For this review, take the finished solid that the model builds, in its own axes (mm). Give positions to 0.01 mm unless a question says otherwise; leave off trailing zeros. Write each loop counter-clockwise with the first axis right and the second up, starting at its lowest first coordinate (ties: lowest second). Pieces come first, ordered by that corner, then holes.
1) For P1, Ø3, axis at x = 0, z = 142.5, coming from the +Y side; P2, Ø2.5, axis at x = 0, z = 142.5, coming from the -Y side, all flat-tipped, find the tip position at first contact; note any pin that passes through.
2) We need section A-A on z = 57. Give the boundary of the cut face in (x, y), and give its area (3 significant figures).
3) Wall thickness on line 1 along X through (y, z) = (1.2, 67.5); line 2 along X through (y, z) = (-0.75, 127.5); line 3 along Y through (x, z) = (3.25, 81): over which ranges is each line inside the solid? List them lowest first.
from build123d import *

# Parameters (mm, degrees)
EXTRUDE1_DEPTH             = 150
SKETCH2_R                  = 1.2
EXTRUDE2_DEPTH             = 4.8
SKETCH_R                   = 2.1
SKETCH_R_2                 = 1.2
EXTRUDE4_DEPTH             = 2.3
CHAMFER1_SIZE              = 0.2
LPATTERN1_COUNT            = 10
LPATTERN1_PITCH            = 15
CHAMFER1_OF_LPATTERN1_SIZE = 0.2


with BuildPart() as part:
    # Sketch1 → Extrude1 (new body)
    with BuildSketch(Plane.XY):
        with BuildLine():
            Line((-3.3, -2.4), (3.3, -2.4))
            Line((3.3, -2.4), (3.5, -2.2))
            Line((3.5, -2.2), (3.5, 0.106274607))
            ThreePointArc((3.5, 0.106274607), (3.091294745, 0.282570681), (2.840065792, 0.65))
            Line((2.840065792, 0.65), (2.340065792, 0.65))
            Line((2.340065792, 0.65), (2.340065792, 1.15))
            Line((2.340065792, 1.15), (2.840065792, 1.15))
            ThreePointArc((2.840065792, 1.15), (3.091294745, 1.517429319), (3.5, 1.693725393))
            Line((3.5, 1.693725393), (3.5, 2.2))
            Line((3.5, 2.2), (3.3, 2.4))
            Line((3.3, 2.4), (-3.3, 2.4))
            Line((-3.3, 2.4), (-3.5, 2.2))
            Line((-3.5, 2.2), (-3.5, 1.693725393))
            ThreePointArc((-3.5, 1.693725393), (-3.091294745, 1.517429319), (-2.840065792, 1.15))
            Line((-2.840065792, 1.15), (-2.340065792, 1.15))
            Line((-2.340065792, 1.15), (-2.340065792, 0.65))
            Line((-2.340065792, 0.65), (-2.840065792, 0.65))
            ThreePointArc((-2.840065792, 0.65), (-3.091294745, 0.282570681), (-3.5, 0.106274607))
            Line((-3.5, 0.106274607), (-3.5, -2.2))
            Line((-3.5, -2.2), (-3.3, -2.4))
        make_face()
    extrude(amount=EXTRUDE1_DEPTH)

    # Sketch2 → Extrude2 (cut)
    with BuildSketch(Plane(origin=(0, 2.4, 0), x_dir=(1, 0, 0), z_dir=(0, 1, 0))):
        with Locations((0, -7.5)):
            Circle(SKETCH2_R)
    extrude2 = extrude(amount=-EXTRUDE2_DEPTH, mode=Mode.SUBTRACT)

    # Sketch → Extrude4 (cut)
    with BuildSketch(Plane(origin=(0, 2.4, 0), x_dir=(1, 0, 0), z_dir=(0, 1, 0))):
        with Locations((0, -7.5)):
            Circle(SKETCH_R)
        with Locations((0, -7.5)):
            Circle(SKETCH_R_2, mode=Mode.SUBTRACT)
    extrude4 = extrude(amount=-EXTRUDE4_DEPTH, mode=Mode.SUBTRACT)

    # Chamfer1
    chamfer1_edges = [part.edges().sort_by_distance(p)[0] for p in [
        (-1.2, -2.4, 7.5),
        (-2.1, 2.4, 7.5),
    ]]
    chamfer(chamfer1_edges, length=CHAMFER1_SIZE)

    # LPattern1: Extrude2, Extrude4 ×10
    with Locations(*[(0, 0, i * LPATTERN1_PITCH) for i in range(1, LPATTERN1_COUNT)]):
        add(extrude2, mode=Mode.SUBTRACT)
        add(extrude4, mode=Mode.SUBTRACT)

    # Chamfer1 of LPattern1
    chamfer1_of_lpattern1_edges = [part.edges().sort_by_distance(p)[0] for p in [
        (-1.2, -2.4, 22.5),
        (-2.1, 2.4, 22.5),
        (-1.2, -2.4, 37.5),
        (-2.1, 2.4, 37.5),
        (-1.2, -2.4, 52.5),
        (-2.1, 2.4, 52.5),
        (-1.2, -2.4, 67.5),
        (-2.1, 2.4, 67.5),
        (-1.2, -2.4, 82.5),
        (-2.1, 2.4, 82.5),
        (-1.2, -2.4, 97.5),
        (-2.1, 2.4, 97.5),
        (-1.2, -2.4, 112.5),
        (-2.1, 2.4, 112.5),
        (-1.2, -2.4, 127.5),
        (-2.1, 2.4, 127.5),
        (-1.2, -2.4, 142.5),
        (-2.1, 2.4, 142.5),
    ]]
    chamfer(chamfer1_of_lpattern1_edges, length=CHAMFER1_OF_LPATTERN1_SIZE)


solid = part.part
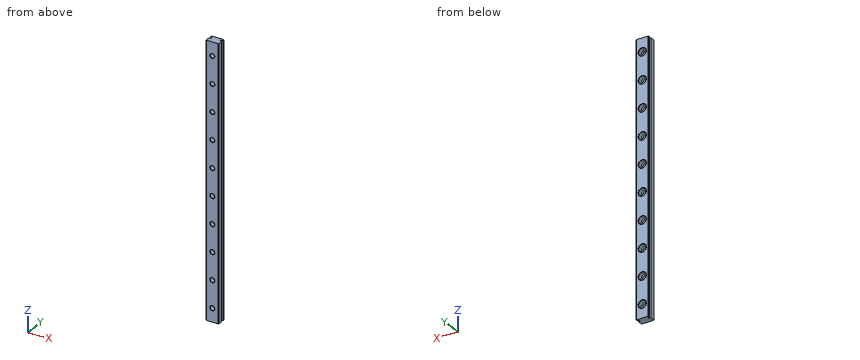
Results list:
1. P1: stops at y = 0.1
1. P2: stops at y = -2.25
2. outline: (-3.5, -2.2) - (-3.3, -2.4) - (3.3, -2.4) - (3.5, -2.2) - (3.5, 0.11) arc R0.8 cw to (2.84, 0.65) - (2.34, 0.65) - (2.34, 1.15) - (2.84, 1.15) arc R0.8 cw to (3.5, 1.69) - (3.5, 2.2) - (3.3, 2.4) - (-3.3, 2.4) - (-3.5, 2.2) - (-3.5, 1.69) arc R0.8 cw to (-2.84, 1.15) - (-2.34, 1.15) - (-2.34, 0.65) - (-2.84, 0.65) arc R0.8 cw to (-3.5, 0.11) - close
2. area: 31.4 mm2
3. line 1: x = -2.86 to -2.1, 2.1 to 2.86
3. line 2: x = -3.5 to -1.2, 1.2 to 3.5
3. line 3: y = -2.4 to 0.18, 1.62 to 2.4
